Study the drawing (mm; zero at the part's minimum x, y, z) and answer. Give positions to 0.01 mm unless a question says otherwise; leave off trailing zeros. Write each loop counter-clockwise with the first axis right and the second up, starting at its lowest first coordinate (ties: lowest second). Pieces come first, ordered by that corner, then holes. Notation, with made-up numbers: (77.25, -22) - (113.25, -22) arc R13 ccw to (113.25, -2) - close; hole circle Ø8 at (-19, -38). An arc over 180 degrees is marked (long way). Answer in a Markdown table with one row per item. Add a question column.
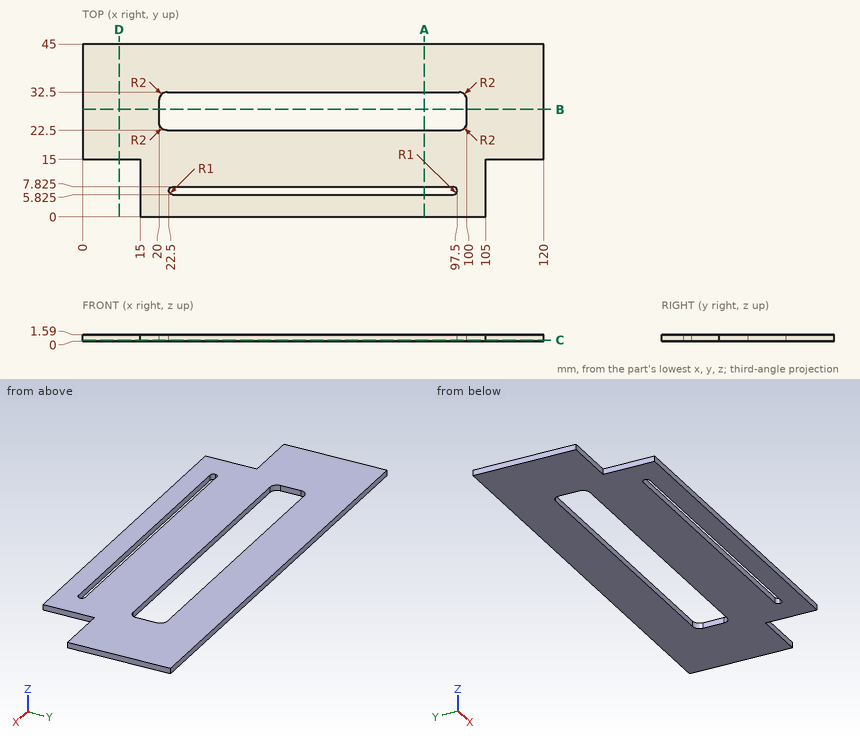
1. Section A-A (x = 89) is taken. Give the vertices of the cut face in (y, z) (3 decimals), and give its area (3 significant figures).
2. Section D-D (x = 9.5) is taken. Give the vertices of the cut face in (y, z), and give its area (3 significant figures).
3. Given pin 1 Ø6 at (x, y) = (32.5, 28) entering from +Z; pin 2 Ø0.5 at (y, z) = (7, 0.5) entering from +X; pin 3 Ø0.8 at (x, z) = (7, 0.5) entering from -Y; pin 4 Ø0.5 at (y, z) = (7.5, 0.5) entering from -X, each flat-ended and moving along its own axis, determine where each tip first touches the part or whether it passes through.
4. Straight lines are drawn through the part: L1, parallel to Y at x = 66, z = 0.35 (3 decimals); L2, parallel to X at y = 29.5, z = 0.6; L3, parallel to X at y = 11, z = 0.2. For each, find the intervals that lie inside material, in ascending order. Write a range as [from, to].
5. Section C-C (z = 0.25) is taken. State how many separate pieces and enclosed holes the cut face has, and give its area (3 significant figures).
6. Section B-B (y = 28) is taken. Give the vertices of the cut face in (x, z).
Geometry check:
| question | item | result |
|---|---|---|
| 1 | outline | (0, 0) - (5.825, 0) - (5.825, 1.59) - (0, 1.59) - close; (7.825, 0) - (22.5, 0) - (22.5, 1.59) - (7.825, 1.59) - close; (32.5, 0) - (45, 0) - (45, 1.59) - (32.5, 1.59) - close |
| 1 | area | 52.5 mm² |
| 2 | outline | (15, 0) - (45, 0) - (45, 1.59) - (15, 1.59) - close |
| 2 | area | 47.7 mm² |
| 3 | pin 1 | through |
| 3 | pin 2 | x = 105 |
| 3 | pin 3 | y = 15 |
| 3 | pin 4 | x = 15 |
| 4 | L1 | [0, 5.825], [7.825, 22.5], [32.5, 45] |
| 4 | L2 | [0, 20], [100, 120] |
| 4 | L3 | [15, 105] |
| 5 | separate pieces | 1 |
| 5 | enclosed holes | 2 |
| 5 | area | 4,000 mm² |
| 6 | outline | (0, 0) - (20, 0) - (20, 1.59) - (0, 1.59) - close; (100, 0) - (120, 0) - (120, 1.59) - (100, 1.59) - close |
